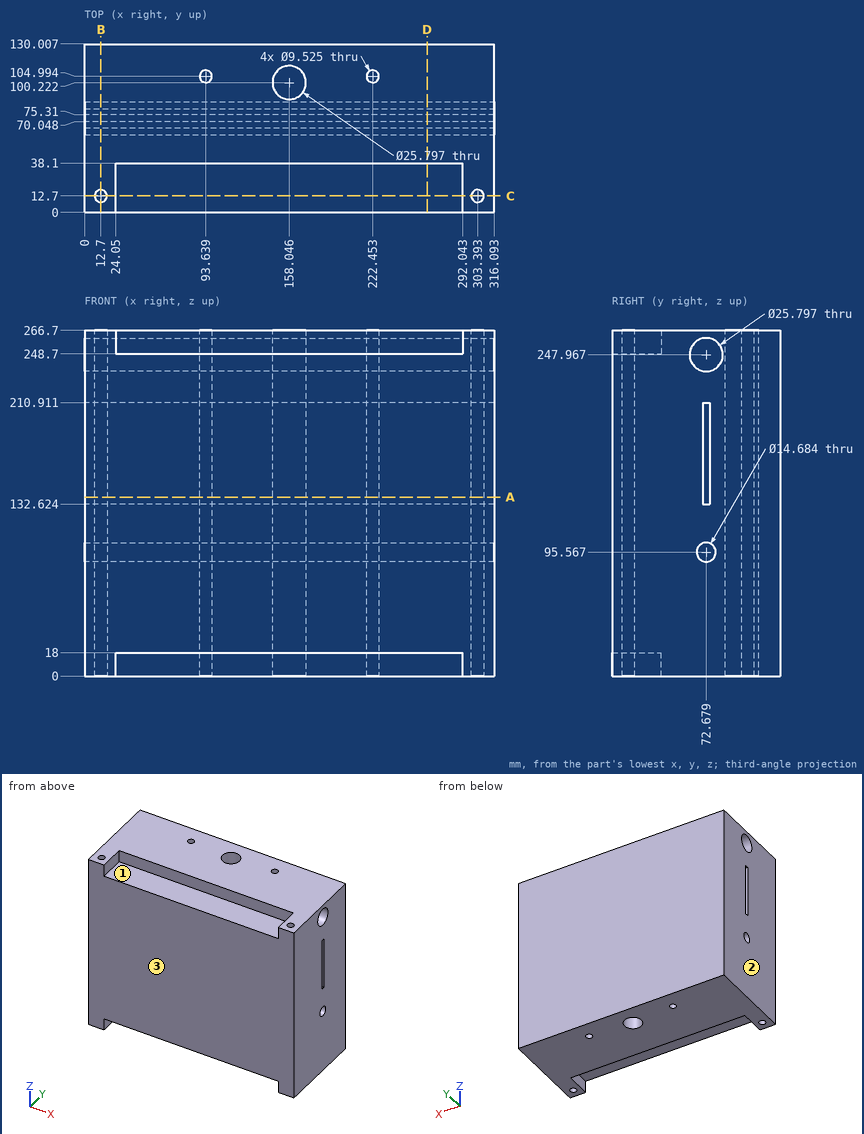
Geometry: see drawing. Coordinates: mm, zero at the bounding-box minimum. Round coordinates to 2 decimals unless told otherwise and drop trailing zeros. Loops run counter-clockwise (first coordinate to the right, second up) from the corner with the lowest first, then second, coordinate; pieces in that order, holes last. Notation, with made-up numbers: (49, 11.25) - (73, 11.25) arc R24 cw to (73, 21.25) - close; hole circle Ø4 at (56.5, 20.5). An arc over 180 degrees is marked (long way). Write item = value, one per line. Start each with the question number.
(1) Section query D-D, the plane x = 264.5. Output: boundary loops of the cut face in (y, z) (1 decimal).
(2) Pull-direction query (X, two-part tool) for the marked faces 1, 2 and 3; classes: +X half, -X half, draft (parallel to the pull), parting line (faces both ways), or undercut.
(3) Ray query, line 1 along Y through (x, z) = (40.5, 170.5); line 2 along X through (y, z) = (14, 104) (1 decimal); line 3 along X through (y, z) = (99, 86.5) (1 decimal). Return the intervals inside material, ascending. Write a range as from..to.
(4) Section query A-A, the plane z = 138. Output: boundary loops of the cut face in (x, y) (1 decimal).
(5) Section query C-C, the plane y = 12.7. State how many separate pieces and enclosed holes the cut face has, plus the area to 3 significant figures.
(6) Pin query (flat end, axial travel): pin 1 (5.5 mm diameter, centred on y = 24.5, z = 9.5, fed in from -X); pin 2 (11.5 mm diameter, centred on x = 158.5, y = 17.5, fed in from -Z); pin 3 (5.5 mm diameter, centred on x = 164.5, z = 9, fed in from -Y). Return the tip coordinate at first contact, or that it passes through.
(7) Section query B-B, the plane x = 12.7. Output: boundary loops of the cut face in (y, z) (1 decimal), plus the area to 3 significant figures.
Conclusion:
q1.outline = (0, 18) - (38.1, 18) - (38.1, 0) - (130, 0) - (130, 266.7) - (38.1, 266.7) - (38.1, 248.7) - (0, 248.7) - close; hole circle Ø25.8 at (72.7, 248); hole circle Ø14.7 at (72.7, 95.6); hole (70, 132.6) - (75.3, 132.6) - (75.3, 210.9) - (70, 210.9) - close
q2.face_1 = undercut
q2.face_2 = -X half
q2.face_3 = draft
q3.line_1 = 0..70.05, 75.31..130.01
q3.line_2 = 0..8.1, 17.3..298.8, 308..316.1
q3.line_3 = 0..145.2, 170.9..316.1
q4.outline = (0, 0) - (316.1, 0) - (316.1, 70) - (0, 70) - close; (0, 75.3) - (316.1, 75.3) - (316.1, 130) - (0, 130) - close; hole circle Ø9.5 at (12.7, 12.7); hole circle Ø9.5 at (93.6, 105); hole circle Ø25.8 at (158, 100.2); hole circle Ø9.5 at (222.5, 105); hole circle Ø9.5 at (303.4, 12.7)
q5.separate_pieces = 3
q5.enclosed_holes = 0
q5.area = 69,600 mm2
q6.pin_1 = 0
q6.pin_2 = 18
q6.pin_3 = 38.1
q7.outline = (0, 0) - (7.9, 0) - (7.9, 266.7) - (0, 266.7) - close; (17.5, 0) - (130, 0) - (130, 266.7) - (17.5, 266.7) - close; hole circle Ø25.8 at (72.7, 248); hole circle Ø14.7 at (72.7, 95.6); hole (70, 132.6) - (75.3, 132.6) - (75.3, 210.9) - (70, 210.9) - close
q7.area = 31,000 mm2
